Here's the drawing with two shaded views (mm, measured from the low corner). I have some questions. A direction names the side the tool comes from. Round coordinates to 2 decimals unless told otherwise and drop trailing zeros. Loops run counter-clockwise (first coordinate to the right, second up) from the corner with the lowest first, then second, coordinate; pieces in that order, holes last. Notation, with made-up numbers: (-20, 79.25) - (1, 79.25) arc R30 cw to (1, 105.25) - close; hole circle Ø4 at (38.25, 17). An arc over 180 degrees is marked (long way). Use one line per item in the form item = value.
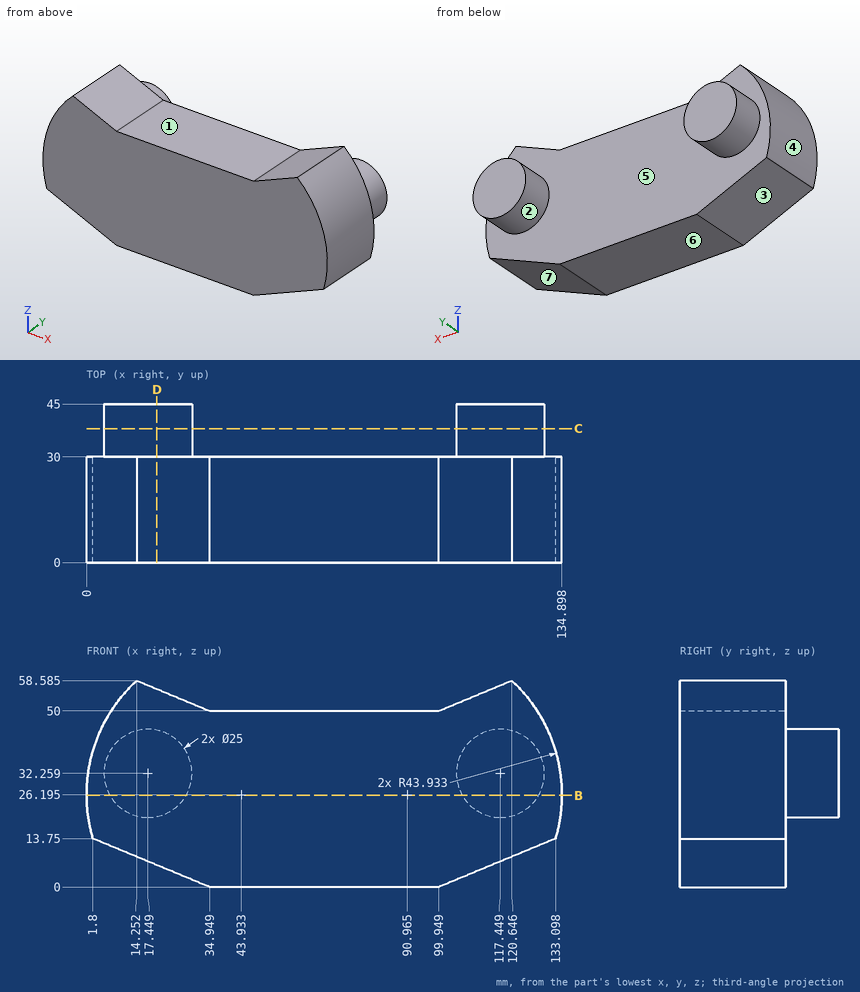
1. We'd pull the mould along X, two halves only. Please class the marked faces 4, 5, 6 and 7: +X half, -X half, draft (parallel to the pull), parting line (faces both ways), or undercut.
Solution:
face_4 = -X half
face_5 = undercut
face_6 = draft
face_7 = +X half
2. If we section it at B-B, the plane z = 26: Write out the boundary of the cut face in (x, y), plus the area to 3 significant figures.
Solution:
outline = (0, 0) - (134.9, 0) - (134.9, 30) - (128.27, 30) - (128.27, 45) - (106.63, 45) - (106.63, 30) - (28.27, 30) - (28.27, 45) - (6.63, 45) - (6.63, 30) - (0, 30) - close
area = 4,700 mm^2
3. For P1, Ø10, axis at x = 100.5, z = 45, coming from the +Y side; P2, Ø10, axis at y = 21.5, z = 33, coming from the +X side; P3, Ø2, axis at y = 21, z = 14, coming from the -X side, each with a flat end and sliding along its axis, tell me the tip position at first contact or that it passes through.
Solution:
P1 = 30
P2 = 134.86
P3 = 1.45
4. On a 3-axis mill with a long thin cutter (end or side, diameter ignored), from which of +Z, -Z, +X, -X, +Y, -Y can I reach the whole of each face in a straight line? I mean the marked faces 1, 2 and 3. Say none if no direction works.
Solution:
face_1 = +Z, +Y, -Y
face_2 = +Y
face_3 = -Z, -X, +Y, -Y
5. If we section it at C-C, the plane y = 38: Write out the boundary of the cut face in (x, z).
Solution:
outline = circle Ø25 at (17.45, 32.26); circle Ø25 at (117.45, 32.26)
6. Please list where these lines run through material, in increasing order: line 1 along Y through (x, z) = (92, 31); line 2 along Z through (x, y) = (85.5, 28); line 3 along X through (y, z) = (17, 55) (1 decimal).
Solution:
line_1 = 0 to 30
line_2 = 0 to 50
line_3 = 10.8 to 22.9, 112 to 124.1
7. If we section it at D-D, the plane x = 20: Write out the boundary of the cut face in (y, z) (1 decimal), plus the area to 3 significant figures.
Solution:
outline = (0, 6.2) - (30, 6.2) - (30, 20) - (45, 20) - (45, 44.5) - (30, 44.5) - (30, 56.2) - (0, 56.2) - close
area = 1,870 mm^2
